The model under review builds one solid part; all positions refer to its coordinate system, in mm. A direction names the side the tool comes from. Coordinates: 2 decimals unless noted, no trailing zeros. Loops run counter-clockwise (first coordinate to the right, second up) from the corner with the lowest first, then second, coordinate; pieces in that order, holes last. Notation, with made-up numbers: M 47,71 L 100,71 A20 cw 100,78 Z; hole C -11.5,46.5 d6. An arc over 180 degrees is marked long. One line per item, written item: value.
```python
from build123d import *

# Parameters (mm, degrees)
F0_R     = 50.8
F0_R_2   = 31.75
F1_DEPTH = 12.7
F2_R     = 2.54
F3_W     = 12.7
F3_H     = 12.7
F4_DEPTH = 2.54


with BuildPart() as f1:
    # F0 (on Front) → F1 (new body)
    with BuildSketch(Plane.XZ):
        Circle(F0_R)
        Circle(F0_R_2, mode=Mode.SUBTRACT)
    extrude(amount=F1_DEPTH)

    # F2
    f2_edges = [f1.edges().sort_by_distance(p)[0] for p in [
        (-50.8, -12.7, 0),
        (-31.75, -12.7, 0),
    ]]
    fillet(f2_edges, radius=F2_R)

    # F3 (on Front) → F4 (join)
    with BuildSketch(Plane.XZ):
        with Locations((0, 44.45)):
            Rectangle(F3_W, F3_H)
    extrude(amount=-F4_DEPTH)


solid = f1.part
```
(1) Insertion check: pin 1 Ø5 at (y, z) = (1, 15.5) entering from -X; pin 2 Ø0.8 at (x, y) = (1.5, 1) entering from -Z; pin 3 Ø6 at (y, z) = (-6.5, 16) entering from +X. Each pin has a flat end and moves straight along its axis. Give the tip position at first contact, or say it passes through.
Checks:
pin 1: x = -49.05
pin 2: z = 38.1
pin 3: x = 49.11
(2) To check wall thickness, follow L1, parallel to Z at x = 0, y = -7; L2, parallel to Y at x = 10, z = 37.5; L3, parallel to X at y = -1.5, z = 15.5. State the ranges of each line that lie inside material, in increasing order. Write a range as [from, to].
Checks:
L1: [-50.8, -31.75], [31.75, 50.8]
L2: [-12.7, 0]
L3: [-48.38, -27.71], [27.71, 48.38]
(3) Add section B-B on y = -1.25. State the section outline as (x, z) points.
Checks:
outline: C 0,0 d101.6; hole C 0,0 d63.5
(4) Tool access review of faces 1 (the face through (6.35, 1, 44)), 2 (the face through (0, 2.54, 45)), 3 (the face through (0, 1, 38.1)): name each direction out of +Z, -Z, +X, -X, +Y, -Y from which nothing blocks a thin tool from reaching the whole face with its end or side.
Checks:
face 1: +Z, -Z, +X, +Y
face 2: +Z, -Z, +X, -X, +Y
face 3: -Z, +X, -X, +Y
(5) Draft analysis for pull direction X (two halves, no side actions). For faces 4 (the face through (-6.883, -5.009, -30.995)), 5 (the face through (-33, -12.7, -10)), 6 (the face through (-6.35, 1, 44)), state which applies: pulls with the +X half, pulls with the -X half, needs draft (parallel to the pull), parting line crosses it, or undercut.
Checks:
face 4: undercut
face 5: needs draft
face 6: pulls with the -X half
(6) Add section A-A on z = 0. State the section outline as (x, y) points, then the cut area to 3 significant figures.
Checks:
outline: M -50.8,-10.16 A2.54 ccw -48.26,-12.7 L -34.29,-12.7 A2.54 ccw -31.75,-10.16 L -31.75,0 L -50.8,0 Z; M 31.75,-10.16 A2.54 ccw 34.29,-12.7 L 48.26,-12.7 A2.54 ccw 50.8,-10.16 L 50.8,0 L 31.75,0 Z
area: 478 mm^2
